Check sheet for the modelled part. Datum: model origin and axes. Units: mm. Give positions to 0.01 mm unless a question says otherwise; leave off trailing zeros. Write each loop counter-clockwise with the first axis right and the second up, starting at its lowest first coordinate (ties: lowest second). Pieces come first, ordered by that corner, then holes. Notation, with made-up numbers: M -20.75,1 L 35.25,1 A9 cw 35.25,8 Z; hole C 35.25,78.25 d2. An arc over 180 degrees is marked long. One line per item, written item: value. Start each with the question number.
from build123d import *

# Parameters (mm, degrees)
EXTRUDE_1_DEPTH     = 3
SKETCH_2_R          = 1.5
CUT_EXTRUDE_1_DEPTH = 10
SKETCH_3_W          = 10
SKETCH_3_H          = 172
SKETCH_3_W_2        = 90
SKETCH_3_H_2        = 33
EXTRUDE_2_DEPTH     = 3
SKETCH_4_R          = 1.5
CUT_EXTRUDE_2_DEPTH = 10
SKETCH_5_R          = 1.5
CUT_EXTRUDE_3_DEPTH = 10
SKETCH_6_R          = 1.5
CUT_EXTRUDE_4_DEPTH = 10
SKETCH_7_R          = 1.5
CUT_EXTRUDE_5_DEPTH = 74
SKETCH_8_R          = 1.5
CUT_EXTRUDE_6_DEPTH = 10
SKETCH_9_W          = 6
SKETCH_9_H          = 172
EXTRUDE_3_DEPTH     = 3
SKETCH_10_R         = 1.5
CUT_EXTRUDE_7_DEPTH = 15
CHAMFER_2_SIZE      = 2.5
CHAMFER_3_SIZE      = 2.5
CHAMFER_4_SIZE      = 2.5
CHAMFER_5_SIZE      = 2.5
CHAMFER_6_SIZE      = 2.5
CHAMFER_7_SIZE      = 2.5
CHAMFER_8_SIZE      = 2.5
SKETCH_11_R         = 1.5
CUT_EXTRUDE_8_DEPTH = 10


with BuildPart() as part:
    # 草图1 → 凸台-拉伸1 (new body)
    with BuildSketch(Plane.XY):
        Polygon((-105.75, 86), (-105.75, 70), (-105.75, -86), (105.75, -86), (105.75, 86), align=None)
    extrude(amount=EXTRUDE_1_DEPTH)

    # 草图2 → 切除-拉伸1 (cut)
    with BuildSketch(Plane.XY.offset(3)):
        with Locations((97.05, 83)):
            Circle(SKETCH_2_R)
        with Locations((-93.55, 83)):
            Circle(SKETCH_2_R)
        with Locations((57.55, 83)):
            Circle(SKETCH_2_R)
        with Locations((-54.05, 83)):
            Circle(SKETCH_2_R)
        with Locations((57.55, -83)):
            Circle(SKETCH_2_R)
        with Locations((97.05, -83)):
            Circle(SKETCH_2_R)
        with Locations((-54.05, -83)):
            Circle(SKETCH_2_R)
        with Locations((-93.55, -83)):
            Circle(SKETCH_2_R)
    extrude(amount=-CUT_EXTRUDE_1_DEPTH, mode=Mode.SUBTRACT)

    # 草图3 → 凸台-拉伸2 (add)
    with BuildSketch(Plane.XY.offset(3)):
        with Locations((110.75, 0)):
            Rectangle(SKETCH_3_W, SKETCH_3_H)
        with Locations((1.75, 99.5)):
            Rectangle(SKETCH_3_W_2, SKETCH_3_H_2)
        with Locations((1.75, -99.5)):
            Rectangle(SKETCH_3_W_2, SKETCH_3_H_2)
    extrude(amount=-EXTRUDE_2_DEPTH)

    # 草图4 → 切除-拉伸2 (cut)
    with BuildSketch(Plane.XY.offset(3)):
        with Locations((44.55, 68)):
            Circle(SKETCH_4_R)
        with Locations((14.55, -14)):
            Circle(SKETCH_4_R)
        with Locations((14.55, 14)):
            Circle(SKETCH_4_R)
        with Locations((44.55, -68)):
            Circle(SKETCH_4_R)
    extrude(amount=-CUT_EXTRUDE_2_DEPTH, mode=Mode.SUBTRACT)

    # 草图5 → 切除-拉伸3 (cut)
    with BuildSketch(Plane.XY.offset(3)):
        with Locations((92.75, 45)):
            Circle(SKETCH_5_R)
        with Locations((92.75, 25)):
            Circle(SKETCH_5_R)
        with Locations((92.75, -25)):
            Circle(SKETCH_5_R)
        with Locations((92.75, -45)):
            Circle(SKETCH_5_R)
    extrude(amount=-CUT_EXTRUDE_3_DEPTH, mode=Mode.SUBTRACT)

    # 草图6 → 切除-拉伸4 (cut)
    with BuildSketch(Plane.XY.offset(3)):
        with Locations((25.25, -89)):
            Circle(SKETCH_6_R)
        with Locations((-21.75, 89)):
            Circle(SKETCH_6_R)
        with Locations((25.25, 89)):
            Circle(SKETCH_6_R)
        with Locations((-21.75, -89)):
            Circle(SKETCH_6_R)
    extrude(amount=-CUT_EXTRUDE_4_DEPTH, mode=Mode.SUBTRACT)

    # 草图7 → 切除-拉伸5 (cut)
    with BuildSketch(Plane(origin=(0, 0, 0), x_dir=(-1, 0, 0), z_dir=(0, 0, -1))):
        with Locations((91.75, -60)):
            Circle(SKETCH_7_R)
        with Locations((91.75, -40)):
            Circle(SKETCH_7_R)
        with Locations((91.75, 60)):
            Circle(SKETCH_7_R)
        with Locations((91.75, 40)):
            Circle(SKETCH_7_R)
    extrude(amount=-CUT_EXTRUDE_5_DEPTH, mode=Mode.SUBTRACT)

    # 草图8 → 切除-拉伸6 (cut)
    with BuildSketch(Plane(origin=(0, 0, 0), x_dir=(-1, 0, 0), z_dir=(0, 0, -1))):
        with Locations((-97.75, 10)):
            Circle(SKETCH_8_R)
        with Locations((-97.75, -10)):
            Circle(SKETCH_8_R)
    extrude(amount=-CUT_EXTRUDE_6_DEPTH, mode=Mode.SUBTRACT)

    # 草图9 → 凸台-拉伸3 (add)
    with BuildSketch(Plane(origin=(0, 0, 0), x_dir=(-1, 0, 0), z_dir=(0, 0, -1))):
        with Locations((108.75, 0)):
            Rectangle(SKETCH_9_W, SKETCH_9_H)
    extrude(amount=-EXTRUDE_3_DEPTH)

    # 草图10 → 切除-拉伸7 (cut)
    with BuildSketch(Plane(origin=(0, 0, 0), x_dir=(-1, 0, 0), z_dir=(0, 0, -1))):
        with Locations((105.75, 76)):
            Circle(SKETCH_10_R)
        with Locations((105.75, 25)):
            Circle(SKETCH_10_R)
        with Locations((105.75, -25)):
            Circle(SKETCH_10_R)
        with Locations((105.75, -76)):
            Circle(SKETCH_10_R)
    extrude(amount=-CUT_EXTRUDE_7_DEPTH, mode=Mode.SUBTRACT)

    # 倒角2
    chamfer_2_edges = [part.edges().sort_by_distance(p)[0] for p in [
        (23.75, 89, 0),
    ]]
    chamfer(chamfer_2_edges, length=CHAMFER_2_SIZE)

    # 倒角3
    chamfer_3_edges = [part.edges().sort_by_distance(p)[0] for p in [
        (-23.25, 89, 0),
        (-90.25, -60, 0),
        (-90.25, -40, 0),
        (-90.25, 60, 0),
        (-90.25, 40, 0),
        (-104.25, 76, 0),
        (-104.25, 25, 0),
        (-104.25, -25, 0),
        (-104.25, -76, 0),
    ]]
    chamfer(chamfer_3_edges, length=CHAMFER_3_SIZE)

    # 倒角4
    chamfer_4_edges = [part.edges().sort_by_distance(p)[0] for p in [
        (43.05, -68, 0),
        (23.75, -89, 0),
        (-23.25, -89, 0),
    ]]
    chamfer(chamfer_4_edges, length=CHAMFER_4_SIZE)

    # 倒角5
    chamfer_5_edges = [part.edges().sort_by_distance(p)[0] for p in [
        (91.25, 45, 0),
        (91.25, 25, 0),
        (91.25, -25, 0),
        (91.25, -45, 0),
        (99.25, 10, 0),
        (99.25, -10, 0),
    ]]
    chamfer(chamfer_5_edges, length=CHAMFER_5_SIZE)

    # 倒角6
    chamfer_6_edges = [part.edges().sort_by_distance(p)[0] for p in [
        (13.05, 14, 0),
    ]]
    chamfer(chamfer_6_edges, length=CHAMFER_6_SIZE)

    # 倒角7
    chamfer_7_edges = [part.edges().sort_by_distance(p)[0] for p in [
        (43.05, 68, 0),
    ]]
    chamfer(chamfer_7_edges, length=CHAMFER_7_SIZE)

    # 倒角8
    chamfer_8_edges = [part.edges().sort_by_distance(p)[0] for p in [
        (13.05, -14, 0),
    ]]
    chamfer(chamfer_8_edges, length=CHAMFER_8_SIZE)

    # 草图11 → 切除-拉伸8 (cut)
    with BuildSketch(Plane(origin=(0, 0, 0), x_dir=(-1, 0, 0), z_dir=(0, 0, -1))):
        with Locations((-89.209242617, 70.25)):
            Circle(SKETCH_11_R)
        with Locations((-99.209242617, 70.25)):
            Circle(SKETCH_11_R)
    cut_extrude_8 = extrude(amount=-CUT_EXTRUDE_8_DEPTH, mode=Mode.SUBTRACT)

    # 镜向1: 切除-拉伸8 across plane
    add(cut_extrude_8.mirror(Plane.ZX), mode=Mode.SUBTRACT)


solid = part.part
1) Cross-section at A-A (z = 0.8). State how many separate pieces and enclosed holes the cut face has, plus the area to 3 significant figures.
2) Material ranges on L1, parallel to X at y = 89, z = 2.7; L2, parallel to X at y = 83, z = 0.8; L3, parallel to X at y = -76, z = 2.8, recorded low to high. Write a range as from..to.
3) Draft check along X on faces 1 (the conical face through (-107.248, 24.379, 2.379)), 2 (the flat face through (4, 2, 0)). Enter one of: released by +X, released by -X, zero draft, split by the parting line, or undercut.
4) Cross-section at B-B (x = -80.5). Record the boundary of the cut face in (y, z), plus the area to 3 significant figures.
5) Gauge pin test, flat ends, axial feed: pin 1 (5 mm diameter, centred on x = 14.55, y = -14, fed in from -Z); pin 2 (0.9 mm diameter, centred on y = -103.5, z = 2, fed in from -X). Record the tip position at first contact, or that the pin passes through.
Data:
1. separate pieces: 1
1. enclosed holes: 34
1. area: 43,700 mm2
2. L1: x = -43.25..-23.25, -20.25..23.75, 26.75..46.75
2. L2: x = -111.75..-95.05, -92.05..-55.55, -52.55..56.05, 59.05..95.55, 98.55..115.75
2. L3: x = -111.75..-107.25, -104.25..115.75
3. face 1: undercut
3. face 2: zero draft
4. outline: M -86,0 L 86,0 L 86,3 L -86,3 Z
4. area: 516 mm2
5. pin 1: stops at z = 1.5
5. pin 2: stops at x = -43.25
